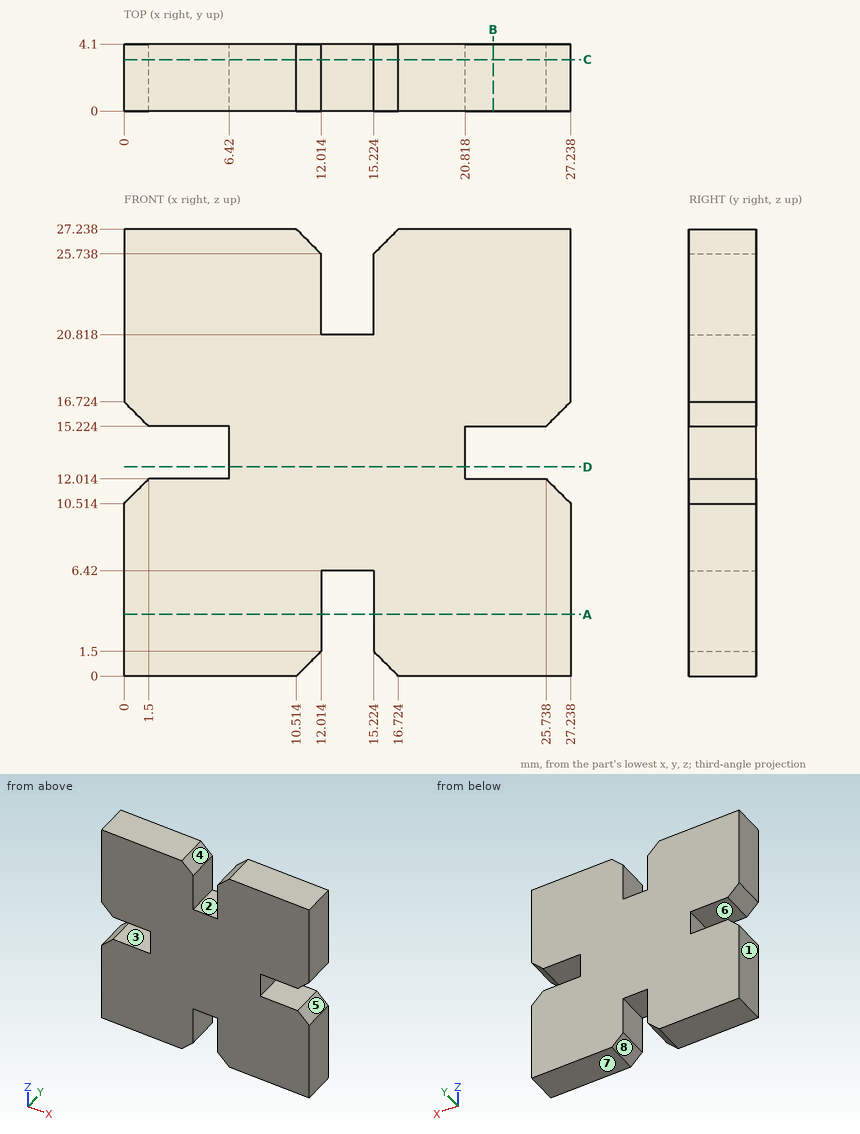
Design review of the part shown in the three views and the two pictorial views. Dimensions are in mm from the part's minimum x, y and z. A direction names the side the tool comes from. Round coordinates to 2 decimals unless told otherwise and drop trailing zeros. Loops run counter-clockwise (first coordinate to the right, second up) from the corner with the lowest first, then second, coordinate; pieces in that order, holes last. Notation, with made-up numbers: M 43,52.25 L 74,52.25 A17 cw 74,82.25 Z; hole C 25.25,21 d11. An arc over 180 degrees is marked long. Answer as a JSON object with one key per item and string values.
Item 1: We need section A-A on z = 3.75. Give the boundary of the cut face in (x, y).
Answer sheet:
{"outline": "M 0,0 L 12.01,0 L 12.01,4.1 L 0,4.1 Z; M 15.22,0 L 27.24,0 L 27.24,4.1 L 15.22,4.1 Z"}
Item 2: Machinability: for the marked faces 4, 5, 6, 7 and 8, which of the approach directions +Z, -Z, +X, -X, +Y, -Y give a long, thin tool a straight path to every point of the face, cutting with its end or side? Answer none if there is none.
Answer sheet:
{"face 4": "+Z, +Y, -Y", "face 5": "+X, +Y, -Y", "face 6": "-X, +Y, -Y", "face 7": "-Z, +X, -X, +Y, -Y", "face 8": "-Z, +Y, -Y"}
Item 3: We need section B-B on x = 22.5. Give the boundary of the cut face in (y, z), and give its area (3 significant figures).
Answer sheet:
{"outline": "M 0,0 L 4.1,0 L 4.1,12.01 L 0,12.01 Z; M 0,15.22 L 4.1,15.22 L 4.1,27.24 L 0,27.24 Z", "area": "98.5 mm^2"}
Item 4: Wall thickness on L1, parallel to X at y = 3.4, z = 24.75; L2, parallel to Z at x = 14.5, y = 0.85: over which ranges is each line inside the solid? List them lowest first. Write a range as from..to.
Answer sheet:
{"L1": "x = 0..12.01, 15.22..27.24", "L2": "z = 6.42..20.82"}
Item 5: We need section C-C on y = 3.15. Give the boundary of the cut face in (x, z).
Answer sheet:
{"outline": "M 0,0 L 10.51,0 L 12.01,1.5 L 12.01,6.42 L 15.22,6.42 L 15.22,1.5 L 16.72,0 L 27.24,0 L 27.24,10.51 L 25.74,12.01 L 20.82,12.01 L 20.82,15.22 L 25.74,15.22 L 27.24,16.72 L 27.24,27.24 L 16.72,27.24 L 15.22,25.74 L 15.22,20.82 L 12.01,20.82 L 12.01,25.74 L 10.51,27.24 L 0,27.24 L 0,16.72 L 1.5,15.22 L 6.42,15.22 L 6.42,12.01 L 1.5,12.01 L 0,10.51 Z"}
Item 6: The part is to be moulded in two halves that separate along X. For the marked faces 1, 2 and 3, say which applies: pulls with the +X half, pulls with the -X half, needs draft (parallel to the pull), parting line crosses it, or undercut.
Answer sheet:
{"face 1": "pulls with the -X half", "face 2": "undercut", "face 3": "needs draft"}
Item 7: Clearance check with flat-ended pins moving along their axes: P1, Ø1.6, axis at y = 2, z = 14, coming from the +X side; P2, Ø2, axis at x = 5, y = 3, coming from the -Z side; P3, Ø1.6, axis at x = 14.5, y = 1, coming from the -Z side. State where each tip first meets the part, or that it passes through.
Answer sheet:
{"P1": "stops at x = 20.82", "P2": "stops at z = 0", "P3": "stops at z = 1.42"}
Item 8: We need section D-D on z = 12.75. Give the boundary of the cut face in (x, y), and give its area (3 significant figures).
Answer sheet:
{"outline": "M 6.42,0 L 20.82,0 L 20.82,4.1 L 6.42,4.1 Z", "area": "59.0 mm^2"}
